The listing builds one solid part. Answer for the finished solid, in the listing's coordinates (mm). A direction names the side the tool comes from. Round coordinates to 2 decimals unless told otherwise and drop trailing zeros. Loops run counter-clockwise (first coordinate to the right, second up) from the corner with the lowest first, then second, coordinate; pieces in that order, holes last. Notation, with made-up numbers: M 36,-33 L 91,-33 A25 ccw 91,-5 Z; hole C 8,-11 d4. An arc over 180 degrees is marked long. Answer as a JSON object with one key per item and string values.
```python
from build123d import *

# Parameters (mm, degrees)
BOSS_EXTRUDE1_DEPTH = 10
CUT_EXTRUDE1_DEPTH  = 10


with BuildPart() as part:
    # Sketch1 → Boss-Extrude1 (new body)
    with BuildSketch(Plane.XY):
        with BuildLine():
            Line((-3.862051717, 61.551449242), (3.862051717, 61.551449242))
            Line((3.862051717, 61.551449242), (9.267481785, 49.133631876))
            ThreePointArc((9.267481785, 49.133631876), (12.940952255, 48.296291314), (16.540941283, 47.184714278))
            Line((16.540941283, 47.184714278), (27.431089723, 55.236144542))
            Line((27.431089723, 55.236144542), (34.120359519, 51.374092825))
            Line((34.120359519, 51.374092825), (32.592690593, 37.917232493))
            ThreePointArc((32.592690593, 37.917232493), (35.355339059, 35.355339059), (37.917232493, 32.592690593))
            Line((37.917232493, 32.592690593), (51.374092825, 34.120359519))
            Line((51.374092825, 34.120359519), (55.236144542, 27.431089723))
            Line((55.236144542, 27.431089723), (47.184714278, 16.540941283))
            ThreePointArc((47.184714278, 16.540941283), (48.296291314, 12.940952255), (49.133631876, 9.267481785))
            Line((49.133631876, 9.267481785), (61.551449242, 3.862051717))
            Line((61.551449242, 3.862051717), (61.551449242, -3.862051717))
            Line((61.551449242, -3.862051717), (49.133631876, -9.267481785))
            ThreePointArc((49.133631876, -9.267481785), (48.296291314, -12.940952255), (47.184714278, -16.540941283))
            Line((47.184714278, -16.540941283), (55.236144542, -27.431089723))
            Line((55.236144542, -27.431089723), (51.374092825, -34.120359519))
            Line((51.374092825, -34.120359519), (37.917232493, -32.592690593))
            ThreePointArc((37.917232493, -32.592690593), (35.355339059, -35.355339059), (32.592690593, -37.917232493))
            Line((32.592690593, -37.917232493), (34.120359519, -51.374092825))
            Line((34.120359519, -51.374092825), (27.431089723, -55.236144542))
            Line((27.431089723, -55.236144542), (16.540941283, -47.184714278))
            ThreePointArc((16.540941283, -47.184714278), (12.940952255, -48.296291314), (9.267481785, -49.133631876))
            Line((9.267481785, -49.133631876), (3.862051717, -61.551449242))
            Line((3.862051717, -61.551449242), (-3.862051717, -61.551449242))
            Line((-3.862051717, -61.551449242), (-9.267481785, -49.133631876))
            ThreePointArc((-9.267481785, -49.133631876), (-12.940952255, -48.296291314), (-16.540941283, -47.184714278))
            Line((-16.540941283, -47.184714278), (-27.431089723, -55.236144542))
            Line((-27.431089723, -55.236144542), (-34.120359519, -51.374092825))
            Line((-34.120359519, -51.374092825), (-32.592690593, -37.917232493))
            ThreePointArc((-32.592690593, -37.917232493), (-35.355339059, -35.355339059), (-37.917232493, -32.592690593))
            Line((-37.917232493, -32.592690593), (-51.374092825, -34.120359519))
            Line((-51.374092825, -34.120359519), (-55.236144542, -27.431089723))
            Line((-55.236144542, -27.431089723), (-47.184714278, -16.540941283))
            ThreePointArc((-47.184714278, -16.540941283), (-48.296291314, -12.940952255), (-49.133631876, -9.267481785))
            Line((-49.133631876, -9.267481785), (-61.551449242, -3.862051717))
            Line((-61.551449242, -3.862051717), (-61.551449242, 3.862051717))
            Line((-61.551449242, 3.862051717), (-49.133631876, 9.267481785))
            ThreePointArc((-49.133631876, 9.267481785), (-48.296291314, 12.940952255), (-47.184714278, 16.540941283))
            Line((-47.184714278, 16.540941283), (-55.236144542, 27.431089723))
            Line((-55.236144542, 27.431089723), (-51.374092825, 34.120359519))
            Line((-51.374092825, 34.120359519), (-37.917232493, 32.592690593))
            ThreePointArc((-37.917232493, 32.592690593), (-35.355339059, 35.355339059), (-32.592690593, 37.917232493))
            Line((-32.592690593, 37.917232493), (-34.120359519, 51.374092825))
            Line((-34.120359519, 51.374092825), (-27.431089723, 55.236144542))
            Line((-27.431089723, 55.236144542), (-16.540941283, 47.184714278))
            ThreePointArc((-16.540941283, 47.184714278), (-12.940952255, 48.296291314), (-9.267481785, 49.133631876))
            Line((-9.267481785, 49.133631876), (-3.862051717, 61.551449242))
        make_face()
    extrude(amount=BOSS_EXTRUDE1_DEPTH)

    # Sketch2 → Cut-Extrude1 (cut)
    with BuildSketch(Plane(origin=(0, 0, 0), x_dir=(-1, 0, 0), z_dir=(0, 0, -1))):
        with BuildLine():
            Line((3.5, -25), (3.5, -19.691368668))
            ThreePointArc((3.5, -19.691368668), (0, 20), (-3.5, -19.691368668))
            Line((-3.5, -19.691368668), (-3.5, -25))
            Line((-3.5, -25), (0, -25))
            Line((0, -25), (3.5, -25))
        make_face()
    extrude(amount=-CUT_EXTRUDE1_DEPTH, mode=Mode.SUBTRACT)


solid = part.part
```
Item 1: Straight lines are drawn through the part: line 1 (X direction, y = 0, z = 3); line 2 (Y direction, x = -10, z = 8); line 3 (X direction, y = -4, z = 0.75). For each, find the intervals that lie inside material, in ascending order.
Values follow:
{"line 1": "-61.55 to -20, 20 to 61.55", "line 2": "-48.99 to -17.32, 17.32 to 48.99", "line 3": "-61.23 to -19.6, 19.6 to 61.23"}
Item 2: The part is cut by section C-C (y = -45.5). Give the vertices of the cut face in (x, z).
Values follow:
{"outline": "M -33.45,0 L 33.45,0 L 33.45,10 L -33.45,10 Z"}
Item 3: Flat-ended cylindrical pins translate along their axes: P1, Ø1, axis at x = 41, z = 4.5, coming from the -Y side; P2, Ø2, axis at y = -39, z = 8.5, coming from the -X side; P3, Ø3, axis at x = 13, z = 6, coming from the -Y side. Find the tip coordinate at first contact, or state that the pin passes through.
Values follow:
{"P1": "y = -33", "P2": "x = -32.83", "P3": "y = -48.66"}
Item 4: The part is cut by section A-A (x = 0). Give the vertices of the cut face in (y, z).
Values follow:
{"outline": "M -61.55,0 L -25,0 L -25,10 L -61.55,10 Z; M 20,0 L 61.55,0 L 61.55,10 L 20,10 Z"}
Item 5: Which of the six approach directions +Z, -Z, +X, -X, +Y, -Y give full straight-line access (tool end or side, diameter ignored) to faces 5 (the face through (12.89, 48.31, 4.93)), 6 (the face through (-48.283, -12.992, 4.93)), 7 (the face through (22.062, -51.267, 4.93)), 8 (the face through (55.429, -6.527, 4.93)), 9 (the face through (3.5, -22, 5))?
Values follow:
{"face 5": "+Z, -Z, +Y", "face 6": "+Z, -Z, -X", "face 7": "+Z, -Z, -Y", "face 8": "+Z, -Z, +X", "face 9": "+Z, -Z"}
Item 6: The part is cut by section B-B (y = 0). Give the vertices of the cut face in (x, z), then the cut area to 3 significant figures.
Values follow:
{"outline": "M -61.55,0 L -20,0 L -20,10 L -61.55,10 Z; M 20,0 L 61.55,0 L 61.55,10 L 20,10 Z", "area": "831 mm^2"}
Item 7: Determine the mould class of faces 1 (the face through (51.154, -21.91, 4.93)), 2 (the face through (15, 15, 10)), 3 (the face through (-22.062, 51.267, 4.93)), 4 (the face through (-55.429, 6.527, 4.93)) for opening direction X: released by +X, released by -X, zero draft, split by the parting line, or undercut.
Values follow:
{"face 1": "released by +X", "face 2": "zero draft", "face 3": "undercut", "face 4": "released by -X"}
